from build123d import *

# Parameters (mm, degrees)
F2_T = -2


# Not quite as in the source:
# - a feature names something its author has since deleted; it is built from what else it names


with BuildPart() as f1:
    # F0 (on Front) → F1 (revolve)
    with BuildSketch(Plane.XZ):
        Polygon((0, -91.5846474071), (0, 63.4153525929), (-80, 63.4153525929), (-80, 18.4153525929), (-77, 18.4153525929), (-50.5, -91.5846474071), align=None)
    revolve(axis=Axis((0, 0, -14.0846474071), (0, 0, -1)))

    # F2
    f2_openings = [f1.faces().sort_by_distance(p)[0] for p in [
        (0, 0, 63.415353),
    ]]
    offset(amount=F2_T, openings=f2_openings, kind=Kind.INTERSECTION)


solid = f1.part
Could you check a few things on this model? Use its own coordinates, in mm. A direction names the side the tool comes from. Coordinates: 2 decimals unless noted, no trailing zeros. Loops run counter-clockwise (first coordinate to the right, second up) from the corner with the lowest first, then second, coordinate; pieces in that order, holes last. Notation, with made-up numbers: (-36.5, 25.5) -> (-17.5, 25.5) arc R28 ccw to (-17.5, 59.5) -> close; hole circle Ø5 at (67.25, 84). An arc over 180 degrees is marked (long way). Answer in a Markdown table with one row per item.
(1) Will these pins go through, and if not, where does the flat tip stop? pin 1 Ø12 at (x, z) = (55, -15.5) entering from -Y; pin 2 Ø10 at (y, z) = (-28, -48) entering from +X; pin 3 Ø4 at (x, y) = (24, -10) entering from +Z.
Results found:
| item | result |
|---|---|
| pin 1 | stops at y = -48.68 |
| pin 2 | stops at x = 56.87 |
| pin 3 | stops at z = -89.58 |
(2) If I drill on probe 1 along Y at (x, z) = (0, 49); probe 2 along Z at (x, y) = (-9.5, 39.5); probe 3 along Y at (x, z) = (56, 2), over which ranges is the centre line in solid material (lowest first)?
Results found:
| item | result |
|---|---|
| probe 1 | y = -80 to -78, 78 to 80 |
| probe 2 | z = -91.58 to -89.58 |
| probe 3 | y = -46.9 to -43.63, 43.63 to 46.9 |
(3) Imagine slicing it at C-C (z = -69). List the corners of the cut face in (x, y) for me, plus the area to 3 significant figures.
Results found:
| item | result |
|---|---|
| outline | circle Ø111.88 at (0, 0); hole circle Ø107.77 at (0, 0) |
| area | 710 mm^2 |
(4) Imagine slicing it at A-A (y = 0). List the corners of the cut face in (x, z) for me.
Results found:
| item | result |
|---|---|
| outline | (-80, 18.42) -> (-77, 18.42) -> (-50.5, -91.58) -> (50.5, -91.58) -> (77, 18.42) -> (80, 18.42) -> (80, 63.42) -> (78, 63.42) -> (78, 20.42) -> (75.42, 20.42) -> (48.92, -89.58) -> (-48.92, -89.58) -> (-75.42, 20.42) -> (-78, 20.42) -> (-78, 63.42) -> (-80, 63.42) -> close |
(5) For faces 1 (the face through (41, 64, 20.415)), 2 (the face through (1, 1, -91.585)), which set-ups out of +Z, -Z, +X, -X, +Y, -Y let a thin tool reach every point of the face, with its end or its side?
Results found:
| item | result |
|---|---|
| face 1 | +Z |
| face 2 | -Z, +X, -X, +Y, -Y |
(6) Thinking about a two-plate mould opening in Y: for faces 3 (the face through (12.8, -57.64, -47.58)), 4 (the face through (42, 66, 18.415)), 5 (the face through (-27.97, -53.78, -49.58)), which applies, released by +Y, released by -Y, zero draft, split by the parting line, or undercut?
Results found:
| item | result |
|---|---|
| face 3 | undercut |
| face 4 | zero draft |
| face 5 | split by the parting line |
